from build123d import *

# Parameters (mm, degrees)
SKETCH1_W           = 15
SKETCH1_H           = 5
BOSS_EXTRUDE1_DEPTH = 5
FILLET3_R           = 15


with BuildPart() as part:
    # Sketch1 → Boss-Extrude1 (new body)
    with BuildSketch(Plane(origin=(0, 0, 0), x_dir=(1, 0, 0), z_dir=(0, 1, 0))):
        Polygon((-34, -25), (-37, -25), (-37, 37.5), (-87, 37.5), (-87, 50), (-19, 50), (-19, -30), (-34, -30), align=None)
        with Locations((-69.5, 42.5)):
            Rectangle(SKETCH1_W, SKETCH1_H, mode=Mode.SUBTRACT)
        with Locations((-44.5, 42.5)):
            Rectangle(SKETCH1_W, SKETCH1_H, mode=Mode.SUBTRACT)
    extrude(amount=BOSS_EXTRUDE1_DEPTH)

    # Fillet3
    fillet3_edges = [part.edges().sort_by_distance(p)[0] for p in [
        (-19, 2.5, -50),
    ]]
    fillet(fillet3_edges, radius=FILLET3_R)


solid = part.part
Source: CAD feature listing. Evaluate the final solid. Frame: model axes, mm. A direction names the side the tool comes from. Coordinates: 2 decimals unless noted, no trailing zeros. Order: outer loops, then holes, each group sorted by start corner. A loop starts at its lowest first (then second) coordinate and runs counter-clockwise, first axis right, second up. Notation, with made-up numbers: M 0,31.25 L 7,31.25 A22 cw 7,57.25 Z; hole C -32,4.25 d1. An arc over 180 degrees is marked long. Write each question's results on one line, items separated by ' | '. Start each with the question number.
Item 1: Cut plane D-D (x = -60). Return loops of the section in (y, z).
Item 2: Cut plane C-C (z = -7). Return loops of the section in (x, y), and give its area (3 significant figures).
Item 3: Cut plane A-A (y = 3.9). Return loops of the section in (x, z).
Item 4: Line query: probe 1 along Z at (x, y) = (-65, 3.75); probe 2 along X at (y, z) = (2.4, 10.5); probe 3 along Z at (x, y) = (-56.5, 3.3). Output: solid intervals per line, ascending.
Item 5: First-contact query: pin 1 Ø1.5 at (y, z) = (0.5, 14) entering from -X; pin 2 Ø1.5 at (x, y) = (-70.5, 1.5) entering from +Z; pin 3 Ø0.9 at (x, y) = (-35, 3.5) entering from +Z. Flat tips, straight axial feed; report the tip coordinate or a pass-through.
Item 6: Draft query along Z for faces 4 (the face through (-34, 2, 28)), 5 (the face through (-45, 2, -40)), 6 (the face through (-23.28, 2.54, -45.49)). Return one class per face: pulls with the +Z half, pulls with the -Z half, needs draft (parallel to the pull), parting line crosses it, or undercut.
Item 7: Set-up query: faces 1 (the face through (-62, 2, -42)), 2 (the face through (-35, 2, 25)), 3 (the face through (-35, 5, -19)). Return all of +Z, -Z, +X, -X, +Y, -Y with unobstructed straight access to the full face (end or side cutting, diameter ignored); none if empty.
Item 8: Cut plane B-B (x = -40). Return loops of the section in (y, z), and give its area (3 significant figures).
Checked values:
1) outline: M 0,-50 L 5,-50 L 5,-37.5 L 0,-37.5 Z
2) outline: M -37,0 L -19,0 L -19,5 L -37,5 Z | area: 90.0 mm2
3) outline: M -87,-50 L -34,-50 A15 ccw -19,-35 L -19,30 L -34,30 L -34,25 L -37,25 L -37,-37.5 L -87,-37.5 Z; hole M -77,-45 L -62,-45 L -62,-40 L -77,-40 Z; hole M -52,-45 L -37,-45 L -37,-40 L -52,-40 Z
4) probe 1: z = -50 to -45, -40 to -37.5 | probe 2: x = -37 to -19 | probe 3: z = -50 to -37.5
5) pin 1: stops at x = -37 | pin 2: stops at z = -37.5 | pin 3: stops at z = 25
6) face 4: needs draft | face 5: undercut | face 6: pulls with the -Z half
7) face 1: +Y, -Y | face 2: +Z, -X, +Y, -Y | face 3: +Z, -Z, +X, -X, +Y
8) outline: M 0,-50 L 5,-50 L 5,-45 L 0,-45 Z; M 0,-40 L 5,-40 L 5,-37.5 L 0,-37.5 Z | area: 37.5 mm2
